Could you check a few things on this model? Use its own coordinates, in mm. Round coordinates to 2 decimals unless told otherwise and drop trailing zeros. Loops run counter-clockwise (first coordinate to the right, second up) from the corner with the lowest first, then second, coordinate; pieces in that order, holes last. Notation, with made-up numbers: (59, 2.5) - (76, 2.5) arc R20 cw to (76, 30.5) - close; hole circle Ø10 at (-2, -16). An arc over 180 degrees is marked (long way). Answer as CSV lines item,"result". Start each with the question number.
1) Suppose I cut it at C-C, the plane z = 4.25. Write out the boundary of the cut face in (x, y).
2) Suppose I cut it at D-D, the plane z = 1.5. Write out the boundary of the cut face in (x, y).
3) Suppose I cut it at A-A, the plane x = 0. Write out the boundary of the cut face in (y, z).
4) Please list where these lines run through material, in increasing order: line 1 along Y through (x, z) = (0.25, 6.5); line 2 along X through (y, z) = (0, 2.5); line 3 along Z through (x, y) = (7, -1.5).
5) I'm going to push flat-ended pins straight in: pin 1 Ø1 at (x, z) = (3, 5.5) entering from -Y; pin 2 Ø1 at (x, z) = (2.5, 5.5) entering from +Y. Where does each tip first touch, or does it pass through?
6) We'd pull the mould along Y, two halves only. Please class faces 1 (the face through (-2.52, 0.33, 3.26)), 2 (the face through (-7.287, -5.587, 6.102)), 3 (the face through (-2, -2, 6.604)): pulls with the +Y half, pulls with the -Y half, needs draft (parallel to the pull), parting line crosses it, or undercut.
Autodesk Inventor part; units mm, degrees
ref_plane "YZ Plane" through (0, 0, 0) normal (1, 0, 0) x (0, 1, 0)
ref_plane "XZ Plane" through (0, 0, 0) normal (0, 1, 0) x (-1, 0, 0)
ref_plane "XY Plane" through (0, 0, 0) normal (0, 0, 1) x (1, 0, 0)
sketch "Sketch1" plane through (0, 0, 0) normal (0, 0, 1) x (1, 0, 0)
  circle A0 centre (0, 0) radius 9.1821
  dimension "d0" = 18.3642
extrude "Extrusion1" add sketch "Sketch1" along normal blind 1.016
sketch "Sketch2" plane through (0, 0, 1.016) normal (0, 0, 1) x (1, 0, 0)
  circle A0 centre (0, 0) radius 6.985
  dimension "d3" = 13.97
extrude "Extrusion2" add sketch "Sketch2" along normal blind 2.286
sketch "Sketch3" plane through (0, 0, 3.302) normal (0, 0, 1) x (1, 0, 0)
  point P0 (0, 0)
hole "Hole1" at (0, 0, 3.302) direction (0, 0, -1) diameter 5.08 depth 25.4 tip angle 118
mirror "Mirror1" about plane through (0, 0, 3.302) normal (0, 0, 1) of "Extrusion2", "Extrusion1", "Hole1"
fillet "Fillet1" radius 2.286 2 edges at (-6.985, 0, 1.016) (-6.985, 0, 5.588)
properties part number "pulley alpha"
Filled sheet:
1,outline,"circle Ø14.38 at (0, 0); hole circle Ø5.08 at (0, 0)"
2,outline,"circle Ø15.73 at (0, 0); hole circle Ø5.08 at (0, 0)"
3,outline,"(-9.18, 0) - (-2.54, 0) - (-2.54, 6.6) - (-9.18, 6.6) - (-9.18, 5.59) arc R2.29 cw to (-9.18, 1.02) - close; (2.54, 0) - (9.18, 0) - (9.18, 1.02) arc R2.29 cw to (9.18, 5.59) - (9.18, 6.6) - (2.54, 6.6) - close"
4,line 1,"-9.18 to -2.53, 2.53 to 9.18"
4,line 2,"-7.13 to -2.54, 2.54 to 7.13"
4,line 3,"0 to 2.43, 4.18 to 6.6"
5,pin 1,"y = -8.83"
5,pin 2,"y = 8.96"
6,face 1,"undercut"
6,face 2,"parting line crosses it"
6,face 3,"needs draft"
